Geometry: final body of the model. Coordinates: model frame, mm. A direction names the side the tool comes from. Round coordinates to 2 decimals unless told otherwise and drop trailing zeros. Loops run counter-clockwise (first coordinate to the right, second up) from the corner with the lowest first, then second, coordinate; pieces in that order, holes last. Notation, with made-up numbers: (73.25, -19) -> (120.25, -19) arc R22 cw to (120.25, -10) -> close; hole circle Ø10 at (9, -29). An arc over 180 degrees is marked (long way). Answer in a Markdown table with one row per item.
```python
from build123d import *

# Parameters (mm, degrees)
ESBO_O1_W                = 10
ESBO_O1_H                = 3
ESBO_O1_W_2              = 140
ESBO_O1_H_2              = 70
RESSALTO_EXTRUS_O1_DEPTH = 3
ESBO_O2_W                = 5
ESBO_O2_H                = 10
RESSALTO_EXTRUS_O2_DEPTH = 3


with BuildPart() as part:
    # Esboço1 → Ressalto-extrusão1 (new body)
    with BuildSketch(Plane.XY):
        with Locations((-65, 36.5)):
            Rectangle(ESBO_O1_W, ESBO_O1_H)
        with Locations((65, -36.5)):
            Rectangle(ESBO_O1_W, ESBO_O1_H)
        with Locations((-65, -36.5)):
            Rectangle(ESBO_O1_W, ESBO_O1_H)
        Rectangle(ESBO_O1_W_2, ESBO_O1_H_2)
        with Locations((65, 36.5)):
            Rectangle(ESBO_O1_W, ESBO_O1_H)
    extrude(amount=RESSALTO_EXTRUS_O1_DEPTH)

    # Esboço2 → Ressalto-extrusão2 (add)
    with BuildSketch(Plane.XY.offset(3)):
        with Locations((-72.5, -30)):
            Rectangle(ESBO_O2_W, ESBO_O2_H)
        with Locations((-72.5, -10)):
            Rectangle(ESBO_O2_W, ESBO_O2_H)
        with Locations((-72.5, 10)):
            Rectangle(ESBO_O2_W, ESBO_O2_H)
        with Locations((-72.5, 30)):
            Rectangle(ESBO_O2_W, ESBO_O2_H)
        with Locations((72.5, 30)):
            Rectangle(ESBO_O2_W, ESBO_O2_H)
        with Locations((72.5, 10)):
            Rectangle(ESBO_O2_W, ESBO_O2_H)
        with Locations((72.5, -10)):
            Rectangle(ESBO_O2_W, ESBO_O2_H)
        with Locations((72.5, -30)):
            Rectangle(ESBO_O2_W, ESBO_O2_H)
    extrude(amount=-RESSALTO_EXTRUS_O2_DEPTH)


solid = part.part
```
Item 1: Mould query, pull axis Y, two halves, no side actions, for faces 4 (the flat face through (-1, 35, 1)), 5 (the flat face through (72, -5, 2)), 6 (the flat face through (75, 30, 2)). Classes: released by +Y, released by -Y, zero draft, split by the parting line, or undercut.
Ans:
| item | result |
|---|---|
| face 4 | released by +Y |
| face 5 | undercut |
| face 6 | zero draft |
Item 2: Section query B-B, the plane y = 17. Output: boundary loops of the cut face in (x, z), and give its area (3 significant figures).
Ans:
| item | result |
|---|---|
| outline | (-70, 0) -> (70, 0) -> (70, 3) -> (-70, 3) -> close |
| area | 420 mm2 |
Item 3: Section query A-A, the plane x = 14. Output: boundary loops of the cut face in (y, z), and give its area (3 significant figures).
Ans:
| item | result |
|---|---|
| outline | (-35, 0) -> (35, 0) -> (35, 3) -> (-35, 3) -> close |
| area | 210 mm2 |
Item 4: First-contact query: P1, Ø1, axis at x = -41, y = -11, coming from the -Z side; P2, Ø0.9, axis at x = 17, z = 1.5, coming from the -Y side; P3, Ø1.5, axis at x = 1.5, z = 0.5, coming from the +Y side; P4, Ø0.9, axis at y = 37, z = 2, coming from the -X side. Flat tips, straight axial feed; report the tip coordinate or a pass-through.
Ans:
| item | result |
|---|---|
| P1 | z = 0 |
| P2 | y = -35 |
| P3 | y = 35 |
| P4 | x = -70 |
Item 5: Set-up query: faces 1 (the flat face through (-73, -25, 2)), 2 (the flat face through (70, 0, 1)), 3 (the flat face through (72, 35, 2)). Return all of +Z, -Z, +X, -X, +Y, -Y with unobstructed straight access to the full face (end or side cutting, diameter ignored); none if empty.
Ans:
| item | result |
|---|---|
| face 1 | +Z, -Z, -X |
| face 2 | +Z, -Z, +X |
| face 3 | +Z, -Z, +X, +Y |
Item 6: Ray query, L1, parallel to Y at x = 42.5, z = 1.9; L2, parallel to X at y = -20.5, z = 0.7. Return the intervals inside material, ascending.
Ans:
| item | result |
|---|---|
| L1 | -35 to 35 |
| L2 | -70 to 70 |
